Build history of the part. All positions in model axes, mm. Face numbers are marked on the shaded views. A direction names the side the tool comes from. Give positions to 0.01 mm unless a question says otherwise; leave off trailing zeros. Order: outer loops, then holes, each group sorted by start corner. A loop starts at its lowest first (then second) coordinate and runs counter-clockwise, first axis right, second up. Notation, with made-up numbers: (19.5, -16.75) - (59.5, -16.75) arc R26 cw to (59.5, 6.25) - close; hole circle Ø2 at (53.25, 81). An arc over 180 degrees is marked (long way). Write each question's results on one line, items separated by ' | '. Start each with the question number.
1) Cut at C-C on y = -8.25. List the corners of the cut face in (x, z), plus the area to 3 significant figures.
2) Tool access for the marked faces 1, 2, 3 and 4: list every direction of +Z, -Z, +X, -X, +Y, -Y with a clear straight run to the whole face (end or side of a thin tool).
3) Drill centre lines: line 1 along Y through (x, z) = (85.6, -13.15); line 2 along Y through (x, z) = (84.65, -12.85); line 3 along Y through (x, z) = (86.5, -9.95). Where is each one in solid material? Low to high. Write a range as from..to.
4) Cut at A-A on z = -10.05. List the corners of the cut face in (x, y).
5) Cut at B-B on y = -14.5. List the corners of the cut face in (x, z).
6) Drop flat-ended pins along their axis: pin 1 Ø0.8 at (x, z) = (85.5, -11) entering from +Y; pin 2 Ø1.5 at (x, z) = (86.5, -13) entering from +Y; pin 3 Ø1 at (x, y) = (86, -3) entering from -Z. Give the stop position or say it passes through.
7) Two-plate mould, pull along Y, no slides. Class the marked faces 5, 6, 7 and 8: +Y half, -Y half, draft (parallel to the pull), parting line (faces both ways), or undercut.
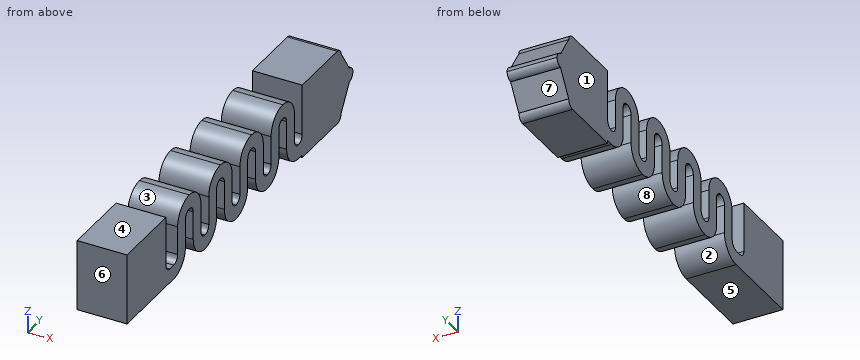
from build123d import *

# Parameters (mm, degrees)
AUFSATZ_LINEAR_AUSTRAGEN3_DEPTH = 2.8
VERRUNDUNG2_R                   = 0.4
VERRUNDUNG5_R                   = 1.2
VERRUNDUNG6_R                   = 1.2
LINEARES_MUSTER1_COUNT          = 5
LINEARES_MUSTER1_PITCH          = 3.2
SKIZZE5_W                       = 4
SKIZZE5_H                       = 4
SKIZZE5_W_2                     = 4.2
AUFSATZ_LINEAR_AUSTRAGEN4_DEPTH = 2.8
VERRUNDUNG3_R                   = 0.4
VERRUNDUNG4_R                   = 0.4
VERRUNDUNG8_R                   = 1.2
FASE1_START                     = 84.3
FASE1_DEPTH                     = 2.8


with BuildPart() as part:
    # Aufsatz-Linear austragen3: read off the stored shape, not the designer's step
    # Aufsatz-Linear austragen3 outline → Aufsatz-Linear austragen3 (new body)
    with BuildSketch(Plane(origin=(84.3, 0, 0), x_dir=(0, 0, -1), z_dir=(1, 0, 0))):
        Polygon((11.9, 5.1), (11.9, 6.3), (11.1, 6.3), (11.1, 4.3), (12.7, 4.3), (12.7, 3.5), (9.5, 3.5), (9.5, 1.1), (12.7, 1.1), (12.7, -0.1), (13.5, -0.1), (13.5, 1.9), (10.3, 1.9), (10.3, 2.7), (13.5, 2.7), (13.5, 5.1), align=None)
    extrude(amount=AUFSATZ_LINEAR_AUSTRAGEN3_DEPTH)

    # Verrundung2
    verrundung2_edges = [part.edges().sort_by_distance(p)[0] for p in [
        (85.7, 1.9, -10.3),
        (85.7, 2.7, -10.3),
        (85.7, 3.5, -12.7),
        (85.7, 4.3, -12.7),
        (85.7, 6.3, -11.1),
        (85.7, 6.3, -11.9),
        (85.7, 1.1, -12.7),
    ]]
    fillet(verrundung2_edges, radius=VERRUNDUNG2_R - 0.0001)  # a hair under: the kernel refuses the full size


with BuildPart() as body_2:
    # Abspalten1: the piece on the far side of the plane
    add(part.part)
    split(bisect_by=Plane.ZX.offset(3.5), keep=Keep.BOTTOM)

    # Verrundung5
    verrundung5_edges = [body_2.edges().sort_by_distance(p)[0] for p in [
        (85.7, 1.1, -9.5),
        (85.7, 3.5, -9.5),
    ]]
    fillet(verrundung5_edges, radius=VERRUNDUNG5_R - 0.0001)  # a hair under: the kernel refuses the full size


with BuildPart() as part_1:
    add(part.part)

    # Abspalten1
    split(bisect_by=Plane.ZX.offset(3.5), keep=Keep.TOP)

    # Verrundung6
    verrundung6_edges = [part_1.edges().sort_by_distance(p)[0] for p in [
        (85.7, 5.1, -13.5),
    ]]
    fillet(verrundung6_edges, radius=VERRUNDUNG6_R)


with BuildPart() as lineares_muster1_1:
    # Lineares Muster1: pattern copy
    add(body_2.part.moved(Location(Vector(0, -1, 0) * (1 * LINEARES_MUSTER1_PITCH))))


with BuildPart() as lineares_muster1_2:
    # Lineares Muster1: pattern copy
    add(body_2.part.moved(Location(Vector(0, -1, 0) * (2 * LINEARES_MUSTER1_PITCH))))


with BuildPart() as lineares_muster1_3:
    # Lineares Muster1: pattern copy
    add(body_2.part.moved(Location(Vector(0, -1, 0) * (3 * LINEARES_MUSTER1_PITCH))))


with BuildPart() as lineares_muster1_4:
    # Lineares Muster1: pattern copy
    add(body_2.part.moved(Location(Vector(0, -1, 0) * (4 * LINEARES_MUSTER1_PITCH))))

    # Skizze5 → Aufsatz-Linear austragen4 (add)
    with BuildSketch(Plane(origin=(84.3, 0, 0), x_dir=(0, 0, -1), z_dir=(1, 0, 0))):
        with Locations((11.5, -14.9)):
            Rectangle(SKIZZE5_W, SKIZZE5_H)
        with Locations((11.55, 3.1)):
            Rectangle(SKIZZE5_W_2, SKIZZE5_H)
    extrude(amount=AUFSATZ_LINEAR_AUSTRAGEN4_DEPTH)


with BuildPart() as aufsatz_linear_austragen4_piece_1:
    # of the separate pieces the step leaves, piece 1, a body of its own (aufsatz_linear_austragen4_pieces)
    add(lineares_muster1_4.part.solids().sort_by_distance((84.3, -9.3, -10.6999))[0])

    # Verrundung3
    verrundung3_edges = [aufsatz_linear_austragen4_piece_1.edges().sort_by_distance(p)[0] for p in [
        (85.7, -12.9, -12.7),
    ]]
    fillet(verrundung3_edges, radius=VERRUNDUNG3_R)


with BuildPart() as aufsatz_linear_austragen4_piece_2:
    # of the separate pieces the step leaves, piece 2, a body of its own (aufsatz_linear_austragen4_pieces)
    add(lineares_muster1_4.part.solids().sort_by_distance((84.3, 1.1, -9.45))[0])


with BuildPart() as part_2:
    add(part_1.part)

    # Kombinieren1: union body 2, Lineares Muster1_1, Lineares Muster1_2, Lineares Muster1_3, Aufsatz-Linear austragen4 piece 1, Aufsatz-Linear austragen4 piece 2
    add(body_2.part)
    add(lineares_muster1_1.part)
    add(lineares_muster1_2.part)
    add(lineares_muster1_3.part)
    add(aufsatz_linear_austragen4_piece_1.part)
    add(aufsatz_linear_austragen4_piece_2.part)

    # Verrundung4
    verrundung4_edges = [part_2.edges().sort_by_distance(p)[0] for p in [
        (85.7, -9.3, -12.7),
        (85.7, -6.1, -12.7),
        (85.7, -2.9, -12.7),
        (85.7, 0.3, -12.7),
        (85.7, 5.1, -9.45),
        (85.7, 5.1, -13.65),
    ]]
    fillet(verrundung4_edges, radius=VERRUNDUNG4_R)

    # Verrundung8
    verrundung8_edges = [part_2.edges().sort_by_distance(p)[0] for p in [
        (85.7, -0.5, -13.5),
        (85.7, -3.7, -13.5),
        (85.7, -1.3, -13.5),
        (85.7, -6.9, -13.5),
        (85.7, -4.5, -13.5),
        (85.7, -10.1, -13.5),
        (85.7, -7.7, -13.5),
        (85.7, -10.9, -13.5),
    ]]
    fillet(verrundung8_edges, radius=VERRUNDUNG8_R - 0.0001)  # a hair under: the kernel refuses the full size

    # Fase1: read off the stored shape, not the designer's step
    # Fase1 outline → Fase1 (add)
    with BuildSketch(Plane.YZ.offset(FASE1_START)):
        with BuildLine():
            ThreePointArc((5.9, -11.1), (5.922012566, -11.100606151), (5.943958417, -11.102422765))
            Line((5.943958417, -11.102422765), (5.098633526, -9.816964992))
            ThreePointArc((5.098633526, -9.816964992), (5.099658235, -9.833468371), (5.1, -9.85))
            Line((5.1, -9.85), (5.1, -11.1))
            Line((5.1, -11.1), (5.9, -11.1))
        make_face()
        with BuildLine():
            Line((5.099976744, -13.254313255), (5.945017032, -11.897458761))
            ThreePointArc((5.945017032, -11.897458761), (5.922544351, -11.899364185), (5.9, -11.9))
            Line((5.9, -11.9), (5.1, -11.9))
            Line((5.1, -11.9), (5.1, -13.25))
            ThreePointArc((5.1, -13.25), (5.099994186, -13.252156659), (5.099976744, -13.254313255))
        make_face()
    extrude(amount=FASE1_DEPTH)


solid = part_2.part
Results:
1) outline: (84.3, -13.31) - (87.1, -13.31) - (87.1, -9.97) - (84.3, -9.97) - close | area: 9.36 mm^2
2) face 1: +Z, -Z, -X, +Y, -Y | face 2: -Z, +X, -X | face 3: +Z, +X, -X | face 4: +Z, +X, -X, -Y
3) line 1: -16.9..-11.25, -9.75..-8.05, -6.55..-4.85, -3.35..-1.65, -0.15..5.16 | line 2: -16.9..-11.03, -9.97..-7.83, -6.77..-4.63, -3.57..-1.43, -0.37..5.35 | line 3: -16.9..-12.9, -11.44..-9.56, -8.24..-6.36, -5.04..-3.16, -1.84..0.04, 1.1..5.19
4) outline: (84.3, -16.9) - (87.1, -16.9) - (87.1, -12.9) - (84.3, -12.9) - close; (84.3, -11.51) - (87.1, -11.51) - (87.1, -9.49) - (84.3, -9.49) - close; (84.3, -8.31) - (87.1, -8.31) - (87.1, -6.29) - (84.3, -6.29) - close; (84.3, -5.11) - (87.1, -5.11) - (87.1, -3.09) - (84.3, -3.09) - close; (84.3, -1.91) - (87.1, -1.91) - (87.1, 0.11) - (84.3, 0.11) - close; (84.3, 1.1) - (87.1, 1.1) - (87.1, 5.25) - (84.3, 5.25) - close
5) outline: (84.3, -13.5) - (87.1, -13.5) - (87.1, -9.5) - (84.3, -9.5) - close
6) pin 1: y = 6.29 | pin 2: y = 5.73 | pin 3: z = -13.5
7) face 5: draft | face 6: -Y half | face 7: +Y half | face 8: undercut
